```python
from build123d import *

# Parameters (mm, degrees)
ESQUISSE1_W                  = 35
ESQUISSE1_H                  = 35
BOSS_EXTRU_1_DEPTH           = 2
ESQUISSE2_R                  = 1.75
ESQUISSE2_W                  = 35
ESQUISSE2_H                  = 1.064971157
ENL_V_MAT_EXTRU_1_DEPTH      = 2
BOSS_EXTRU_2_DEPTH           = 280
ESQUISSE5_W                  = 7
ESQUISSE5_H                  = 6
ESQUISSE5_R                  = 1.75
BOSS_EXTRU_3_DEPTH           = 2
ESQUISSE6_R                  = 1.75
BOSS_EXTRU_4_DEPTH           = 2
ESQUISSE10_W                 = 35
ESQUISSE10_H                 = 33.935028843
ESQUISSE10_R                 = 1.75
BOSS_EXTRU_5_DEPTH           = 2
ESQUISSE15_R                 = 6.5
ESQUISSE15_R_2               = 1.75
ENL_V_MAT_EXTRU_2_DEPTH      = 373
CONG_1_R                     = 2
CONG_2_R                     = 4
ESQUISSE17_R                 = 1.75
BOSS_EXTRU_6_DEPTH           = 2
ENL_V_MAT_EXTRU_3_DEPTH      = 2
ENL_V_MAT_EXTRU_4_DEPTH      = 279
ENL_V_MAT_EXTRU_4_DEPTH_BACK = 391
ESQUISSE20_W                 = 15.34314575
ESQUISSE20_H                 = 24.213203648
ENL_V_MAT_EXTRU_5_DEPTH      = 20
ESQUISSE23_R                 = 2.1
ENL_V_MAT_EXTRU_6_DEPTH      = 10


with BuildPart() as part:
    # Esquisse1 → Boss.-Extru.1 (new body)
    with BuildSketch(Plane(origin=(0, 0, 0), x_dir=(1, 0, 0), z_dir=(0, 1, 0))):
        with Locations((17.5, -17.5)):
            Rectangle(ESQUISSE1_W, ESQUISSE1_H)
    extrude(amount=BOSS_EXTRU_1_DEPTH)

    # Esquisse2 → Enlèv. mat.-Extru.1 (cut)
    with BuildSketch(Plane(origin=(0, 2, 0), x_dir=(1, 0, 0), z_dir=(0, 1, 0))):
        with Locations(Location((30.935029054, -4.064971369, 0), (0, 0, 270))):
            Circle(ESQUISSE2_R)
        with Locations(Location((30.935028843, -30.935028843, 0), (0, 0, 270))):
            Circle(ESQUISSE2_R)
        with Locations(Location((4.064971369, -4.064970946, 0), (0, 0, 270))):
            Circle(ESQUISSE2_R)
        with Locations(Location((4.064971157, -30.935028843, 0), (0, 0, 270))):
            Circle(ESQUISSE2_R)
        with Locations((17.5, -34.467514421)):
            Rectangle(ESQUISSE2_W, ESQUISSE2_H)
    extrude(amount=-ENL_V_MAT_EXTRU_1_DEPTH, mode=Mode.SUBTRACT)

    # Esquisse4 → Boss.-Extru.2 (add)
    with BuildSketch(Plane(origin=(0, 2, 0), x_dir=(1, 0, 0), z_dir=(0, 1, 0))):
        Polygon((17.5, -33.935028843), (7, -33.935028843), (7, -4.064970946), (28, -4.064970946), (28, -33.935028843), align=None)
    extrude(amount=BOSS_EXTRU_2_DEPTH)

    # Esquisse5 → Boss.-Extru.3 (add)
    # profile 1 of 4: a face of its own
    with BuildSketch(Plane.XY.offset(33.935028843)):
        with Locations((31.5, 254)):
            Rectangle(ESQUISSE5_W, ESQUISSE5_H)
        with Locations((31.5, 254)):
            Circle(ESQUISSE5_R, mode=Mode.SUBTRACT)
    # profile 2 of 4: a face of its own
    with BuildSketch(Plane.XY.offset(33.935028843)):
        with Locations((3.5, 254)):
            Rectangle(ESQUISSE5_W, ESQUISSE5_H)
        with Locations((3.5, 254)):
            Circle(ESQUISSE5_R, mode=Mode.SUBTRACT)
    # profile 3 of 4: a face of its own
    with BuildSketch(Plane.XY.offset(33.935028843)):
        with Locations((31.5, 28)):
            Rectangle(ESQUISSE5_W, ESQUISSE5_H)
        with Locations((31.5, 28)):
            Circle(ESQUISSE5_R, mode=Mode.SUBTRACT)
    # profile 4 of 4: a face of its own
    with BuildSketch(Plane.XY.offset(33.935028843)):
        with Locations((3.5, 28)):
            Rectangle(ESQUISSE5_W, ESQUISSE5_H)
        with Locations((3.5, 28)):
            Circle(ESQUISSE5_R, mode=Mode.SUBTRACT)
    extrude(amount=-BOSS_EXTRU_3_DEPTH)

    # Esquisse6 → Boss.-Extru.4 (add)
    # profile 1 of 2: a face of its own
    with BuildSketch(Plane.XY.offset(33.935028843)):
        Polygon((7, 144), (0, 144), (0, 141), (0, 138), (7, 138), (7, 141), align=None)
        with Locations((3.5, 141)):
            Circle(ESQUISSE6_R, mode=Mode.SUBTRACT)
    # profile 2 of 2: a face of its own
    with BuildSketch(Plane.XY.offset(33.935028843)):
        Polygon((35, 144), (28, 144), (28, 141), (28, 138), (35, 138), (35, 141), align=None)
        with Locations((31.5, 141)):
            Circle(ESQUISSE6_R, mode=Mode.SUBTRACT)
    extrude(amount=-BOSS_EXTRU_4_DEPTH)

    # Esquisse10 → Boss.-Extru.5 (add)
    with BuildSketch(Plane(origin=(0, 282, 0), x_dir=(1, 0, 0), z_dir=(0, 1, 0))):
        with Locations((17.5, -16.967514422)):
            Rectangle(ESQUISSE10_W, ESQUISSE10_H)
        with Locations(Location((30.935028843, -30.935028843, 0), (0, 0, 270))):
            Circle(ESQUISSE10_R, mode=Mode.SUBTRACT)
        with Locations(Location((30.935028631, -4.064970946, 0), (0, 0, 270.000013863))):
            Circle(ESQUISSE10_R, mode=Mode.SUBTRACT)
        with Locations(Location((4.064970946, -4.064971369, 0), (0, 0, 270.000013863))):
            Circle(ESQUISSE10_R, mode=Mode.SUBTRACT)
        with Locations(Location((4.064971157, -30.935028843, 0), (0, 0, 270))):
            Circle(ESQUISSE10_R, mode=Mode.SUBTRACT)
    extrude(amount=-BOSS_EXTRU_5_DEPTH)

    # Esquisse15 → Enlèv. mat.-Extru.2 (cut)
    with BuildSketch(Plane(origin=(0, 282, 0), x_dir=(1, 0, 0), z_dir=(0, 1, 0))):
        with Locations(Location((17.5, -17.5, 0), (0, 0, 270))):
            Circle(ESQUISSE15_R)
        with Locations(Location((30.935029054, -4.064971369, 0), (0, 0, 270))):
            Circle(ESQUISSE15_R_2)
    extrude(amount=-ENL_V_MAT_EXTRU_2_DEPTH, mode=Mode.SUBTRACT)

    # Congé1
    cong_1_edges = [part.edges().sort_by_distance(p)[0] for p in [
        (0, 31, 32.935028843),
        (0, 25, 32.935028843),
        (0, 144, 32.935028843),
        (0, 138, 32.935028843),
        (35, 144, 32.935028843),
        (35, 138, 32.935028843),
        (35, 257, 32.935028843),
        (35, 251, 32.935028843),
        (0, 251, 32.935028843),
        (0, 257, 32.935028843),
        (35, 31, 32.935028843),
        (35, 25, 32.935028843),
    ]]
    fillet(cong_1_edges, radius=CONG_1_R)

    # Congé2
    cong_2_edges = [part.edges().sort_by_distance(p)[0] for p in [
        (35, 281, 0),
        (0, 281, 0),
        (0, 1, 0),
        (35, 1, 0),
    ]]
    fillet(cong_2_edges, radius=CONG_2_R)

    # Esquisse17 → Boss.-Extru.6 (add)
    # profile 1 of 4: a face of its own
    with BuildSketch(Plane.XY.offset(33.935028843)):
        with BuildLine():
            Line((0, 148), (0, 146))
            ThreePointArc((0, 146), (0.585786438, 144.585786438), (2, 144))
            Line((2, 144), (7, 144))
            Line((7, 144), (7, 150))
            Line((7, 150), (2, 150))
            ThreePointArc((2, 150), (0.585786438, 149.414213562), (0, 148))
        make_face()
        with Locations((3.5, 147)):
            Circle(ESQUISSE17_R, mode=Mode.SUBTRACT)
    # profile 2 of 4: a face of its own
    with BuildSketch(Plane.XY.offset(33.935028843)):
        with BuildLine():
            Line((0, 136), (0, 134))
            ThreePointArc((0, 134), (0.585786438, 132.585786438), (2, 132))
            Line((2, 132), (7, 132))
            Line((7, 132), (7, 138))
            Line((7, 138), (2, 138))
            ThreePointArc((2, 138), (0.585786438, 137.414213562), (0, 136))
        make_face()
        with Locations((3.5, 135)):
            Circle(ESQUISSE17_R, mode=Mode.SUBTRACT)
    # profile 3 of 4: a face of its own
    with BuildSketch(Plane.XY.offset(33.935028843)):
        with BuildLine():
            ThreePointArc((35, 134), (34.414213562, 132.585786438), (33, 132))
            Line((33, 132), (28, 132))
            Line((28, 132), (28, 138))
            Line((28, 138), (33, 138))
            ThreePointArc((33, 138), (34.414213562, 137.414213562), (35, 136))
            Line((35, 136), (35, 134))
        make_face()
        with Locations((31.5, 135)):
            Circle(ESQUISSE17_R, mode=Mode.SUBTRACT)
    # profile 4 of 4: a face of its own
    with BuildSketch(Plane.XY.offset(33.935028843)):
        with BuildLine():
            ThreePointArc((35, 146), (34.414213562, 144.585786438), (33, 144))
            Line((33, 144), (28, 144))
            Line((28, 144), (28, 150))
            Line((28, 150), (33, 150))
            ThreePointArc((33, 150), (34.414213562, 149.414213562), (35, 148))
            Line((35, 148), (35, 146))
        make_face()
        with Locations((31.5, 147)):
            Circle(ESQUISSE17_R, mode=Mode.SUBTRACT)
    extrude(amount=-BOSS_EXTRU_6_DEPTH)

    # Esquisse18 → Enlèv. mat.-Extru.3 (cut)
    with BuildSketch(Plane.XY.offset(33.935028843)):
        Polygon((2, 138), (7, 138), (7, 144), (2, 144), (-2.362534847, 144), (-2.362534847, 138), align=None)
        Polygon((37.362534847, 138), (33, 138), (28, 138), (28, 144), (33, 144), (37.362534847, 144), align=None)
    extrude(amount=-ENL_V_MAT_EXTRU_3_DEPTH, mode=Mode.SUBTRACT)

    # Esquisse19 → Enlèv. mat.-Extru.4 (cut, two sides: drawn at the far end of the back side and taken through both)
    with BuildSketch(Plane(origin=(0, 0, 4.064970946), x_dir=(-1, 0, 0), z_dir=(0, 0, -1)).offset(-ENL_V_MAT_EXTRU_4_DEPTH_BACK)):
        Polygon((-28, 141), (-7, 141), (34.536866168, 141), (34.536866168, 293.648195663), (-77.45188643, 293.648195663), (-77.45188643, 143.905659046), align=None)
    extrude(amount=ENL_V_MAT_EXTRU_4_DEPTH + ENL_V_MAT_EXTRU_4_DEPTH_BACK, mode=Mode.SUBTRACT)

    # Esquisse20 → Enlèv. mat.-Extru.5 (cut)
    with BuildSketch(Plane(origin=(0, 141, 0), x_dir=(1, 0, 0), z_dir=(0, 1, 0))):
        with Locations((17.5, -18.999999894)):
            Rectangle(ESQUISSE20_W, ESQUISSE20_H)
    extrude(amount=-ENL_V_MAT_EXTRU_5_DEPTH, mode=Mode.SUBTRACT)

    # Esquisse23 → Enlèv. mat.-Extru.6 (cut)
    with BuildSketch(Plane(origin=(0, 2, 0), x_dir=(1, 0, 0), z_dir=(0, 1, 0))):
        with Locations(Location((30.935028843, -30.935028843, 0), (0, 0, 270))):
            Circle(ESQUISSE23_R)
    extrude(amount=-ENL_V_MAT_EXTRU_6_DEPTH, mode=Mode.SUBTRACT)


solid = part.part
```
CAD build for the part. Positions are in the model's coordinates, mm. A direction names the side the tool comes from. Round coordinates to 2 decimals unless told otherwise and drop trailing zeros. Write each loop counter-clockwise with the first axis right and the second up, starting at its lowest first coordinate (ties: lowest second). Pieces come first, ordered by that corner, then holes. Notation, with made-up numbers: (-28, 48) -> (-5, 48) arc R15 ccw to (-5, 69) -> close; hole circle Ø6 at (-27, 65.25). An arc over 180 degrees is marked (long way). Answer in a Markdown table with one row per item. Add a question column.
Item 1: Mould opens along Z. For faces 1 (the face through (27, 141, 19)), 2 (the face through (17, 131, 6.893)), 3 (the face through (1.141, 1.014, 1.203)) say: pulls with the +Z half, pulls with the -Z half, needs draft (parallel to the pull), parting line crosses it, or undercut.
Item 2: Saw through at C-C, the plane y = 69. Write the cut outline in (x, z).
Item 3: Saw through at B-B, the plane z = 17.5. Write the cut outline in (x, y).
Item 4: Saw through at A-A, the plane x = 17.5. Write the cut outline in (y, z).
Item 5: Drill centre lines: line 1 (Y direction, x = 31.5, z = 32.85); line 2 (X direction, y = 135, z = 32.9); line 3 (X direction, y = 75, z = 17.5). Where is each one in solid material? Low to high. Write a range as from..to.
Item 6: Drop flat-ended pins along their axis: pin 1 Ø5.5 at (x, y) = (3.5, 28) entering from +Z (3 decimals); pin 2 Ø2 at (y, z) = (82, 20.5) entering from -X; pin 3 Ø12.5 at (x, z) = (18.5, 15) entering from +Y; pin 4 Ø3 at (x, y) = (5, 27.5) entering from -Z (3 decimals). Give the stop position or say it passes through.
Item 7: Which spindle directions (+Z, -Z, +X, -X, +Y, -Y) get a long thin tool onto all of the face, cutting with end or side? Do faces 4 (the face through (17.4, 121, 24.2)), 5 (the face through (4.142, 1.014, 29.187)), 6 (the face through (4.142, 1.014, 2.317)), 7 (the face through (5, 136.4, 31.935)), 8 (the face through (30, 136.4, 31.935)). Say none if no direction does.
Findings below:
| question | item | result |
|---|---|---|
| 1 | face 1 | needs draft |
| 1 | face 2 | undercut |
| 1 | face 3 | pulls with the -Z half |
| 2 | outline | (7, 4.06) -> (28, 4.06) -> (28, 33.94) -> (7, 33.94) -> close; hole circle Ø13 at (17.5, 17.5) |
| 3 | outline | (0, 0) -> (11, 0) -> (11, 121) -> (9.83, 121) -> (9.83, 141) -> (7, 141) -> (7, 2) -> (0, 2) -> close; (24, 0) -> (35, 0) -> (35, 2) -> (28, 2) -> (28, 141) -> (25.17, 141) -> (25.17, 121) -> (24, 121) -> close |
| 4 | outline | (0, 0) -> (2, 0) -> (2, 4.06) -> (141, 4.06) -> (141, 6.89) -> (121, 6.89) -> (121, 11) -> (0, 11) -> close; (0, 24) -> (121, 24) -> (121, 31.11) -> (141, 31.11) -> (141, 33.94) -> (0, 33.94) -> close |
| 5 | line 1 | y = 25..26.25, 29.75..31, 132..133.25, 136.75..138 |
| 5 | line 2 | x = 0..1.75, 5.25..29.75, 33.25..35 |
| 5 | line 3 | x = 7..11, 24..28 |
| 6 | pin 1 | stops at z = 33.935 |
| 6 | pin 2 | stops at x = 7 |
| 6 | pin 3 | stops at y = 121 |
| 6 | pin 4 | stops at z = 31.935 |
| 7 | face 4 | +Y |
| 7 | face 5 | -Y |
| 7 | face 6 | +Y, -Y |
| 7 | face 7 | -Z, -X, +Y |
| 7 | face 8 | -Z, +X, +Y |
